Source: CAD feature listing. Evaluate the final solid. Frame: model axes, mm. A direction names the side the tool comes from. Coordinates: 2 decimals unless noted, no trailing zeros. Loops run counter-clockwise (first coordinate to the right, second up) from the corner with the lowest first, then second, coordinate; pieces in that order, holes last. Notation, with made-up numbers: (84, 68) -> (99, 68) arc R21 cw to (99, 92) -> close; hole circle Ø10 at (55.25, -12). An arc over 180 degrees is marked (long way). Answer as CSV lines item,"result".
from build123d import *

# Parameters (mm, degrees)
SKETCH1_W                      = 145
SKETCH1_H                      = 50
BOSS_EXTRUDE1_DEPTH            = 25
CUT_EXTRUDE1_DEPTH             = 81.661329025
CUT_EXTRUDE1_DEPTH_BACK        = 81.661329025
F_12_0_12_DIAMETER_HOLE1_D     = 12
F_12_0_12_DIAMETER_HOLE1_DEPTH = 18
M10_TAPPED_HOLE2_D             = 8.5
M10_TAPPED_HOLE2_DEPTH         = 24.946342369
M10_TAPPED_HOLE2_TIP           = 2.553657631
CHAMFER1_SIZE                  = 1
CHAMFER2_SIZE                  = 1
CHAMFER3_SIZE                  = 1


with BuildPart() as part:
    # Sketch1 → Boss-Extrude1 (new, symmetric)
    with BuildSketch(Plane.XY):
        Rectangle(SKETCH1_W, SKETCH1_H)
    extrude(amount=BOSS_EXTRUDE1_DEPTH, both=True)

    # Sketch2 → Cut-Extrude1 (cut, two sides: drawn at the far end of the back side and taken through both)
    with BuildSketch(Plane.XY.offset(-CUT_EXTRUDE1_DEPTH_BACK)):
        Polygon((-72.5, -10), (-37.5, 25), (-72.5, 25), align=None)
    extrude(amount=CUT_EXTRUDE1_DEPTH + CUT_EXTRUDE1_DEPTH_BACK, mode=Mode.SUBTRACT)

    # Ø12.0 (12) Diameter Hole1
    with Locations(Plane.ZY.offset(72.5)):
        with Locations((0, -5)):
            Hole(F_12_0_12_DIAMETER_HOLE1_D / 2, depth=F_12_0_12_DIAMETER_HOLE1_DEPTH)

    # M10 Tapped Hole2
    with Locations(Plane.ZY.offset(54.5)):
        with Locations((0, -5)):
            Hole(M10_TAPPED_HOLE2_D / 2, depth=M10_TAPPED_HOLE2_DEPTH)
            with Locations((0, 0, -(M10_TAPPED_HOLE2_DEPTH + M10_TAPPED_HOLE2_TIP / 2))):  # 118° drill point
                Cone(0, M10_TAPPED_HOLE2_D / 2, M10_TAPPED_HOLE2_TIP, mode=Mode.SUBTRACT)

    # Chamfer1
    chamfer1_edges = [part.edges().sort_by_distance(p)[0] for p in [
        (-72.5, -17.5, -25),
        (-72.5, -17.5, 25),
        (0, -25, 25),
        (-55, 7.5, -25),
        (-55, 7.5, 25),
        (72.5, 0, 25),
        (0, -25, -25),
        (17.5, 25, -25),
        (72.5, 0, -25),
        (17.5, 25, 25),
    ]]
    chamfer(chamfer1_edges, length=CHAMFER1_SIZE)

    # Chamfer2
    chamfer2_edges = [part.edges().sort_by_distance(p)[0] for p in [
        (72.5, -25, 0),
        (72.5, 25, 0),
    ]]
    chamfer(chamfer2_edges, length=CHAMFER2_SIZE)

    # Chamfer3
    chamfer3_edges = [part.edges().sort_by_distance(p)[0] for p in [
        (-72.5, -25, 0),
    ]]
    chamfer(chamfer3_edges, length=CHAMFER3_SIZE)


solid = part.part
(1) Access query for faces 1 (the flat face through (-1, 0, 25)), 2 (the cylindrical face through (-41.852, -0.786, 0.553)). Directions: +Z, -Z, +X, -X, +Y, -Y. A direction counts if a zero-diameter tool reaches every point of the face in a straight line with its end or side. Return the directions, or none.
Computed values:
face 1,"+Z, +X, -X, +Y, -Y"
face 2,"-X"
(2) Cut plane A-A (z = -11.5). Return the cut outline in (x, y), then the cut area to 3 significant figures.
Computed values:
outline,"(-72.5, -24) -> (-71.5, -25) -> (71.5, -25) -> (72.5, -24) -> (72.5, 24) -> (71.5, 25) -> (-37.5, 25) -> (-72.5, -10) -> close"
area,"6,640 mm^2"
(3) Cut plane B-B (x = -47). Return the cut outline in (y, z).
Computed values:
outline,"(-25, -24) -> (-24, -25) -> (14.09, -25) -> (15.5, -24) -> (15.5, 24) -> (14.09, 25) -> (-24, 25) -> (-25, 24) -> close; hole circle Ø8.5 at (-5, 0)"
(4) Material intervals for L1, parallel to Z at x = -35.75, y = -5; L2, parallel to Z at x = -62, y = -5; L3, parallel to X at y = -9.5, z = 20.5, sorted ascending. Write a range as [from, to].
Computed values:
L1,"[-25, -4.25], [4.25, 25]"
L2,"[-25, -6], [6, 25]"
L3,"[-72, 72.5]"
(5) Pin query (flat end, axial travel): pin 1 Ø12 at (y, z) = (7.5, 8) entering from -X; pin 2 Ø13 at (y, z) = (-7.5, 2) entering from -X; pin 3 Ø5 at (y, z) = (6, 16.5) entering from -X; pin 4 Ø9.5 at (y, z) = (-5, 0) entering from -X. Return the tip coordinate at first contact, or that it passes through.
Computed values:
pin 1,"x = -61"
pin 2,"x = -72.5"
pin 3,"x = -59"
pin 4,"x = -54.5"
(6) Draft query along Y for faces 3 (the cylindrical face through (-61.374, -10.857, 1.301)), 4 (the flat face through (-72.5, -17, 0)), 5 (the flat face through (-55.2, 7.3, -0.3)), 6 (the flat face through (-54.5, -9, -3)). Return one class per face: released by +Y, released by -Y, zero draft, split by the parting line, or undercut.
Computed values:
face 3,"undercut"
face 4,"zero draft"
face 5,"released by +Y"
face 6,"undercut"
